Part model, mm, in its own coordinate system. A direction names the side the tool comes from. Coordinates: 2 decimals unless noted, no trailing zeros. Loops run counter-clockwise (first coordinate to the right, second up) from the corner with the lowest first, then second, coordinate; pieces in that order, holes last. Notation, with made-up numbers: M 63.25,79 L 115.25,79 A27 ccw 115.25,102 Z; hole C 55.5,75.25 d6. An arc over 180 degrees is marked long. Answer as a JSON object with one key per item and string values. Group by question number.
1. Drop flat-ended pins along their axis: pin 1 Ø1 at (x, z) = (-7.5, -15.5) entering from -Y; pin 2 Ø2.5 at (x, y) = (-9.5, -2) entering from +Z; pin 3 Ø1.5 at (y, z) = (-1.5, 5.5) entering from -X. Give the stop position or say it passes through.
2. Drill centre lines: L1, parallel to X at y = -1.4, z = 11; L2, parallel to Z at x = -23, y = -0.15; L3, parallel to Y at x = 31, z = 16. Where is each one in solid material? Low to high.
3. Mould opens along Z. For faces 1 (the face through (31.8, -1, 0)), 2 (the face through (0, -1, 17.8)), 3 (the face through (0, -1, -16.8)), 4 (the face through (0, -1, -17.8)) say: released by +Z, released by -Z, zero draft, split by the parting line, or undercut.
4. Saw through at B-B on y = -2.15. Write the cut outline in (x, z), then the cut area to 3 significant figures.
5. Saw through at C-C on z = -13. Write the cut outline in (x, y), then the cut area to 3 significant figures.
6. 3-axis set-ups, long thin cutter, end or side, ignore diameter. For faces 5 (the face through (-35, 1, 0)), 6 (the face through (32.8, -1, 0)), 7 (the face through (0, -1, 16.8)), 8 (the face through (-32.8, -1, 0)): which of +Z, -Z, +X, -X, +Y, -Y reach the whole face in a straight line?
7. Saw through at A-A on x = 5. Write the cut outline in (y, z), then the cut area to 3 significant figures.
Autodesk Fusion 360 part; units mm, degrees
sketch "Sketch1" plane through (0, 0, 0) normal (0, 1, 0) x (1, 0, 0)
  line L0 (-35, 20) -> (35, 20)
  line L1 (35, 20) -> (35, -20)
  line L2 (35, -20) -> (-35, -20)
  line L3 (-35, -20) -> (-35, 20)
  line L4 (-35, 20) -> (35, -20) construction
  dimension "d106" = 70
  dimension "d107" = 40
extrude "Extrude1" add sketch "Sketch1" along normal blind 2
fillet "Fillet1" radius 3 4 edges at (-35, 1, 20) (35, 1, -20) (-35, 1, -20) (35, 1, 20)
sketch "Sketch2" plane through (0, 0, 0) normal (0, -1, 0) x (1, 0, 0)
  arc A0 (35, 17) -> (32, 20) centre (32, 17) ccw
  line L0 (32, 20) -> (-32, 20)
  arc A1 (-32, 20) -> (-35, 17) centre (-32, 17) ccw
  line L1 (-35, 17) -> (-35, -17)
  arc A2 (-35, -17) -> (-32, -20) centre (-32, -17) ccw
  line L2 (-32, -20) -> (32, -20)
  arc A3 (32, -20) -> (35, -17) centre (32, -17) ccw
  line L3 (35, -17) -> (35, 17)
  line L4 (-32.8, 17) -> (-32.8, -17)
  arc A4 (-32.8, -17) -> (-32, -17.8) centre (-32, -17) ccw
  line L5 (-32, -17.8) -> (32, -17.8)
  arc A5 (32, -17.8) -> (32.8, -17) centre (32, -17) ccw
  line L6 (32.8, -17) -> (32.8, 17)
  arc A6 (32.8, 17) -> (32, 17.8) centre (32, 17) ccw
  line L7 (32, 17.8) -> (-32, 17.8)
  arc A7 (-32, 17.8) -> (-32.8, 17) centre (-32, 17) ccw
  line L8 (-31.8, 16.8) -> (-31.8, -16.8)
  line L9 (-31.8, -16.8) -> (31.8, -16.8)
  line L10 (31.8, -16.8) -> (31.8, 16.8)
  line L11 (31.8, 16.8) -> (-31.8, 16.8)
  dimension "d111" = -2.2
  dimension "d112" = -3.2
extrude "Extrude2" add sketch "Sketch2" along normal blind 3 contours L4 A4 L5 A5 L6 A6 L7 A7
Outcome:
{
 "1": {"pin 1": "stops at y = 0", "pin 2": "stops at z = 17.8", "pin 3": "stops at x = -32.8"},
 "2": {"L1": "x = -32.8 to -31.8, 31.8 to 32.8", "L2": "z = -17.8 to -16.8, 16.8 to 17.8", "L3": "y = 0 to 2"},
 "3": {"face 1": "undercut", "face 2": "released by +Z", "face 3": "undercut", "face 4": "released by -Z"},
 "4": {"outline": "M -32.8,-17 A0.8 ccw -32,-17.8 L 32,-17.8 A0.8 ccw 32.8,-17 L 32.8,17 A0.8 ccw 32,17.8 L -32,17.8 A0.8 ccw -32.8,17 Z; hole M -31.8,-16.8 L 31.8,-16.8 L 31.8,16.8 L -31.8,16.8 Z", "area": "198 mm²"},
 "5": {"outline": "M -35,0 L -32.8,0 L -32.8,-3 L -31.8,-3 L -31.8,0 L 31.8,0 L 31.8,-3 L 32.8,-3 L 32.8,0 L 35,0 L 35,2 L -35,2 Z", "area": "146 mm²"},
 "6": {"face 5": "+Z, -Z, -X, +Y, -Y", "face 6": "+Z, -Z, +X, -Y", "face 7": "-Y", "face 8": "+Z, -Z, -X, -Y"},
 "7": {"outline": "M -3,-17.8 L 0,-17.8 L 0,-20 L 2,-20 L 2,20 L 0,20 L 0,17.8 L -3,17.8 L -3,16.8 L 0,16.8 L 0,-16.8 L -3,-16.8 Z", "area": "86.0 mm²"}
}
